Geometry check sheet. Reference: drawing and pictorial views, mm from the part's lowest x, y, z. Give positions to 0.01 mm unless a question says otherwise; leave off trailing zeros. Order: outer loops, then holes, each group sorted by start corner. A loop starts at its lowest first (then second) coordinate and runs counter-clockwise, first axis right, second up. Notation, with made-up numbers: (1.5, 85) - (42.5, 85) arc R30 cw to (42.5, 113) - close; hole circle Ø5 at (-36.5, 51). An arc over 180 degrees is marked (long way). Answer in a Markdown table with one row per item.
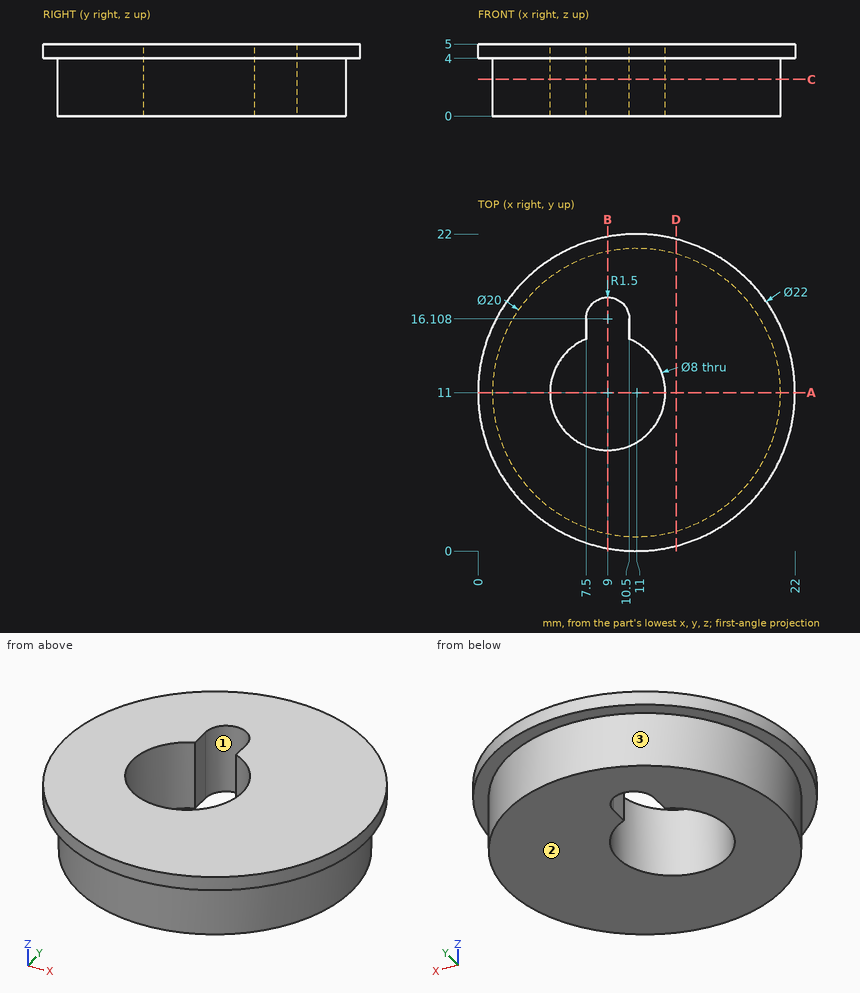
(1) Cross-section at B-B, the plane x = 9. Record the cut outline in (y, z).
Geometry says:
| item | result |
|---|---|
| outline | (0.18, 4) - (1.2, 4) - (1.2, 0) - (7, 0) - (7, 5) - (0.18, 5) - close; (17.61, 0) - (20.8, 0) - (20.8, 4) - (21.82, 4) - (21.82, 5) - (17.61, 5) - close |
(2) Thickness scan on L1, parallel to X at y = 14, z = 4.6; L2, parallel to Y at x = 7.75, z = 3; L3, parallel to Y at x = 5.5, z = 1.7. Record the ranges inside material, lowest first.
Geometry says:
| item | result |
|---|---|
| L1 | 0.42 to 6.35, 11.65 to 21.58 |
| L2 | 1.54 to 7.2, 16.94 to 20.46 |
| L3 | 2.65 to 9.06, 12.94 to 19.35 |
(3) Mould release check, pull along X, two halves, no side actions. Record for the marked faces 1, 2 and 3: pulls with the +X half, pulls with the -X half, needs draft (parallel to the pull), parting line crosses it, or undercut.
Geometry says:
| item | result |
|---|---|
| face 1 | undercut |
| face 2 | needs draft |
| face 3 | parting line crosses it |
(4) Gauge pin test, flat ends, axial feed: P1, Ø3, axis at y = 8.5, z = 0.5, coming from the +X side; P2, Ø1.5, axis at y = 15.5, z = 3.5, coming from the -X side; P3, Ø1.1, axis at y = 15, z = 3, coming from the +X side. Record the tip position at first contact, or that the pin passes through.
Geometry says:
| item | result |
|---|---|
| P1 | x = 20.95 |
| P2 | x = 0.73 |
| P3 | x = 20.39 |
(5) Cross-section at D-D, the plane x = 13.75. Record the cut outline in (y, z), then the cut area to 3 significant figures.
Geometry says:
| item | result |
|---|---|
| outline | (0.35, 4) - (1.39, 4) - (1.39, 0) - (20.61, 0) - (20.61, 4) - (21.65, 4) - (21.65, 5) - (0.35, 5) - close |
| area | 98.2 mm² |
(6) Cross-section at A-A, the plane y = 11. Record the cut outline in (x, z).
Geometry says:
| item | result |
|---|---|
| outline | (0, 4) - (1, 4) - (1, 0) - (5, 0) - (5, 5) - (0, 5) - close; (13, 0) - (21, 0) - (21, 4) - (22, 4) - (22, 5) - (13, 5) - close |
(7) Cross-section at C-C, the plane z = 2.55. Record the cut outline in (x, y).
Geometry says:
| item | result |
|---|---|
| outline | circle Ø20 at (11, 11); hole (7.5, 14.71) arc R4 ccw (long way) to (10.5, 14.71) - (10.5, 16.11) arc R1.5 ccw to (7.5, 16.11) - close |
